```python
from build123d import *

# Parameters (mm, degrees)
SKETCH2_R           = 14.5
SKETCH2_R_2         = 10.5
BOSS_EXTRUDE2_START = -5
SKETCH9_W           = 36
SKETCH9_H           = 36
SKETCH9_R           = 14.5
BOSS_EXTRUDE2_DEPTH = 5
FILLET1_R           = 2
FILLET2_R           = 2
SKETCH10_R          = 3
CUT_EXTRUDE1_DEPTH  = 1
CUT_EXTRUDE2_REACH  = 72.535
SKETCH13_R          = 1.5
CIRPATTERN1_COUNT   = 4
SKETCH15_W          = 36
SKETCH15_H          = 36
SKETCH15_R          = 14.5
BOSS_EXTRUDE6_DEPTH = 5
FILLET3_R           = 2
SKETCH16_R          = 3
CUT_EXTRUDE4_DEPTH  = 1
CUT_EXTRUDE5_REACH  = 86.67
SKETCH17_R          = 1.5
CIRPATTERN2_COUNT   = 4


with BuildPart() as part:
    # Sweep-Thin3: sweep along a path in Sketch1
    with BuildLine(Plane.XY) as sweep_thin3_path:
        Line((0, 0), (-15, 0))
        ThreePointArc((-15, 0), (-33.384776311, 7.615223689), (-41, 26))
        Line((-41, 26), (-41, 41))
    # Sketch2 → Sweep-Thin3 (sweep)
    with BuildSketch(Plane(origin=(0, 0, 0), x_dir=(0, 0, -1), z_dir=(1, 0, 0))):
        Circle(SKETCH2_R)
        Circle(SKETCH2_R_2, mode=Mode.SUBTRACT)
    sweep(path=sweep_thin3_path.line)

    # Sketch9 → Boss-Extrude2 (add)
    with BuildSketch(Plane(origin=(0, 0, 0), x_dir=(0, 0, -1), z_dir=(1, 0, 0)).offset(BOSS_EXTRUDE2_START)):
        Rectangle(SKETCH9_W, SKETCH9_H)
        with Locations(Location((0, 0, 0), (0, 0, 270))):
            Circle(SKETCH9_R, mode=Mode.SUBTRACT)
    extrude(amount=BOSS_EXTRUDE2_DEPTH)

    # Fillet1
    fillet1_edges = [part.edges().sort_by_distance(p)[0] for p in [
        (-2.5, 18, 18),
    ]]
    fillet(fillet1_edges, radius=FILLET1_R)

    # Fillet2
    fillet2_edges = [part.edges().sort_by_distance(p)[0] for p in [
        (-2.5, 18, -18),
        (-2.5, -18, -18),
        (-2.5, -18, 18),
    ]]
    fillet(fillet2_edges, radius=FILLET2_R)

    # Sketch10 → Cut-Extrude1 (cut)
    with BuildSketch(Plane(origin=(0, 0, 0), x_dir=(0, 0, -1), z_dir=(1, 0, 0))):
        with Locations((-13, 13)):
            Circle(SKETCH10_R)
    cut_extrude1 = extrude(amount=-CUT_EXTRUDE1_DEPTH, mode=Mode.SUBTRACT)

    # Sketch13 → Cut-Extrude2 (cut, up to next)
    with BuildSketch(Plane(origin=(-1, 0, 0), x_dir=(0, 0, -1), z_dir=(1, 0, 0)), mode=Mode.PRIVATE) as cut_extrude2_sk1:
        with Locations((-13, 13)):
            Circle(SKETCH13_R)
    cut_extrude2_tool1 = extrude(cut_extrude2_sk1.sketch, amount=-CUT_EXTRUDE2_REACH, mode=Mode.PRIVATE) & part.part
    cut_extrude2 = cut_extrude2_tool1.solids().sort_by_distance((-1, 13, 13))[0]
    add(cut_extrude2, mode=Mode.SUBTRACT)

    # CirPattern1: Cut-Extrude1, Cut-Extrude2 ×4 about axis
    cirpattern1_axis = Axis((0, 0, 0), (1, 0, 0))
    add([cut_extrude1.rotate(cirpattern1_axis, i * 360 / CIRPATTERN1_COUNT) for i in range(1, CIRPATTERN1_COUNT)], mode=Mode.SUBTRACT)
    add([cut_extrude2.rotate(cirpattern1_axis, i * 360 / CIRPATTERN1_COUNT) for i in range(1, CIRPATTERN1_COUNT)], mode=Mode.SUBTRACT)

    # Sketch15 → Boss-Extrude6 (add)
    with BuildSketch(Plane(origin=(0, 41, 0), x_dir=(1, 0, 0), z_dir=(0, 1, 0))):
        with Locations((-41, 0)):
            Rectangle(SKETCH15_W, SKETCH15_H)
        with Locations(Location((-41, 0, 0), (0, 0, 180))):
            Circle(SKETCH15_R, mode=Mode.SUBTRACT)
    extrude(amount=-BOSS_EXTRUDE6_DEPTH)

    # Fillet3
    fillet3_edges = [part.edges().sort_by_distance(p)[0] for p in [
        (-23, 38.5, -18),
        (-23, 38.5, 18),
        (-59, 38.5, 18),
        (-59, 38.5, -18),
    ]]
    fillet(fillet3_edges, radius=FILLET3_R)

    # Sketch16 → Cut-Extrude4 (cut)
    with BuildSketch(Plane(origin=(0, 41, 0), x_dir=(1, 0, 0), z_dir=(0, 1, 0))):
        with Locations(Location((-54, 13, 0), (0, 0, 180))):
            Circle(SKETCH16_R)
    cut_extrude4 = extrude(amount=-CUT_EXTRUDE4_DEPTH, mode=Mode.SUBTRACT)

    # Sketch17 → Cut-Extrude5 (cut, up to next)
    with BuildSketch(Plane(origin=(0, 40, 0), x_dir=(1, 0, 0), z_dir=(0, 1, 0)), mode=Mode.PRIVATE) as cut_extrude5_sk1:
        with Locations(Location((-54, 13, 0), (0, 0, 180))):
            Circle(SKETCH17_R)
    cut_extrude5_tool1 = extrude(cut_extrude5_sk1.sketch, amount=-CUT_EXTRUDE5_REACH, mode=Mode.PRIVATE) & part.part
    cut_extrude5 = cut_extrude5_tool1.solids().sort_by_distance((-54, 40, -13))[0]
    add(cut_extrude5, mode=Mode.SUBTRACT)

    # CirPattern2: Cut-Extrude4, Cut-Extrude5 ×4 about axis
    cirpattern2_axis = Axis((-41, 0, 0), (0, 1, 0))
    add([cut_extrude4.rotate(cirpattern2_axis, i * 360 / CIRPATTERN2_COUNT) for i in range(1, CIRPATTERN2_COUNT)], mode=Mode.SUBTRACT)
    add([cut_extrude5.rotate(cirpattern2_axis, i * 360 / CIRPATTERN2_COUNT) for i in range(1, CIRPATTERN2_COUNT)], mode=Mode.SUBTRACT)


solid = part.part
```
Input: part model. Units: mm. Frame: model coordinates. A direction names the side the tool comes from. Give positions to 0.01 mm unless a question says otherwise; leave off trailing zeros. Write each loop counter-clockwise with the first axis right and the second up, starting at its lowest first coordinate (ties: lowest second). Pieces come first, ordered by that corner, then holes. Notation, with made-up numbers: (84, 60) - (143, 60) arc R14 cw to (143, 77) - close; hole circle Ø4 at (11.25, -7). An arc over 180 degrees is marked (long way). Write item = value, one per line. Start each with the question number.
1) Material intervals for L1, parallel to Y at x = -2, z = -13; L2, parallel to Z at x = -16, y = 0; L3, parallel to Y at x = -26.5, z = -7, sorted ascending. Write a range as [from, to].
2) Cut plane B-B (z = 3). Return loops of the section in (x, y), and give its area (3 significant figures).
3) Cut plane A-A (x = -4). Return loops of the section in (y, z).
4) Cut plane C-C (y = 35). Return loops of the section in (x, z).
5) Reachability of faces 1 (the face through (-55.3, 40, 14.3)), 2 (the face through (-2.97, 13.07, 14.5)), 3 (the face through (-3, 18, 0)), 4 (the face through (-5, 8.3, 12.3)) from +Z, -Z, +X, -X, +Y, -Y: full face, straight path, thin tool, end or side. Return the list, or none.
6) Cut plane D-D (x = -28). Give the number of separate pieces and of enclosed holes in the cut face, and give its area (3 significant figures).
7) Pin query (flat end, axial travel): pin 1 (5 mm diameter, centred on y = 13, z = -13, fed in from +X); pin 2 (8 mm diameter, centred on y = 17, z = -3, fed in from +X); pin 3 (5 mm diameter, centred on y = -13, z = -13, fed in from -X); pin 4 (3 mm diameter, centred on x = -29, z = 12.5, fed in from +Y). Return the tip coordinate at first contact, or that it passes through.
8) Draft query along Y for faces 5 (the face through (-49.3, 36, -12.3)), 6 (the face through (-2.46, -17.4, 17.43)), 7 (the face through (-54.9, 38, 11.8)). Return one class per face: pulls with the +Y half, pulls with the -Y half, needs draft (parallel to the pull), parting line crosses it, or undercut.
Answers follow:
q1.L1 = [-18, -14.5], [-11.5, 11.5], [14.5, 18]
q1.L2 = [-14.5, -10.5], [10.5, 14.5]
q1.L3 = [-10.95, -5.81], [11.93, 19.32], [36, 41]
q2.outline = (-59, 36) - (-55.19, 36) - (-55.19, 26) arc R40.19 ccw to (-15, -14.19) - (-5, -14.19) - (-5, -18) - (0, -18) - (0, -10.06) - (-15, -10.06) arc R36.06 cw to (-51.06, 26) - (-51.06, 41) - (-59, 41) - close; (-30.94, 26) arc R15.94 ccw to (-15, 10.06) - (0, 10.06) - (0, 18) - (-5, 18) - (-5, 14.19) - (-15, 14.19) arc R11.81 cw to (-26.81, 26) - (-26.81, 36) - (-23, 36) - (-23, 41) - (-30.94, 41) - close
q2.area = 661 mm^2
q3.outline = (-18, -16) arc R2 ccw to (-16, -18) - (16, -18) arc R2 ccw to (18, -16) - (18, 16) arc R2 ccw to (16, 18) - (-16, 18) arc R2 ccw to (-18, 16) - close; hole circle Ø3 at (-13, -13); hole circle Ø3 at (-13, 13); hole circle Ø21 at (0, 0); hole circle Ø3 at (13, -13); hole circle Ø3 at (13, 13)
q4.outline = circle Ø29 at (-41, 0); hole circle Ø21 at (-41, 0)
q5.face_1 = +Y
q5.face_2 = +X
q5.face_3 = +Z, -Z, +X, +Y
q5.face_4 = none
q6.separate_pieces = 3
q6.enclosed_holes = 1
q6.area = 716 mm^2
q7.pin_1 = -1
q7.pin_2 = 0
q7.pin_3 = -5
q7.pin_4 = 40
q8.face_5 = undercut
q8.face_6 = pulls with the -Y half
q8.face_7 = needs draft
